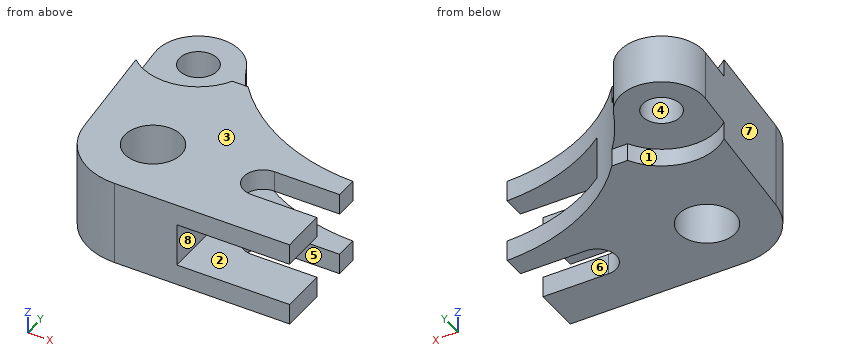
from build123d import *

# Parameters (mm, degrees)
ESQUISSE1_R                  = 9.5
ESQUISSE1_R_2                = 6.35
BOSS_EXTRU_1_DEPTH           = 14.25
ENL_V_MAT_EXTRU_1_DEPTH      = 6
ENL_V_MAT_EXTRU_2_DEPTH      = 7.25
ENL_V_MAT_EXTRU_2_DEPTH_BACK = 7.25


with BuildPart() as part:
    # Esquisse1 → Boss.-Extru.1 (new, symmetric)
    with BuildSketch(Plane.XY):
        with BuildLine():
            Line((-26.61523279, 45.963348263), (-21.894870769, -2.148169925))
            ThreePointArc((-21.894870769, -2.148169925), (-14.777351956, -16.298155392), (0, -22))
            Line((0, -22), (59, -22))
            Line((59, -22), (59, -6.5))
            Line((59, -6.5), (37, -6.5))
            ThreePointArc((37, -6.5), (30.5, 0), (37, 6.5))
            Line((37, 6.5), (59, 6.5))
            Line((59, 6.5), (59, 14))
            ThreePointArc((59, 14), (23.937620364, 25.155899787), (0.053417306, 53.144636986))
            ThreePointArc((0.053417306, 53.144636986), (-16.322360933, 60.848824799), (-26.61523279, 45.963348263))
        make_face()
        with Locations(Location((0, 0, 0), (0, 0, 180))):
            Circle(ESQUISSE1_R, mode=Mode.SUBTRACT)
        with Locations(Location((-12.68213321, 47.330365488, 0), (0, 0, 180))):
            Circle(ESQUISSE1_R_2, mode=Mode.SUBTRACT)
    extrude(amount=BOSS_EXTRU_1_DEPTH, both=True)

    # Esquisse2 → Enlèv. mat.-Extru.1 (cut)
    with BuildSketch(Plane.XY.offset(14.25)):
        with BuildLine():
            Line((4.051067321, 38.330365488), (9.321809703, 38.330365488))
            ThreePointArc((9.321809703, 38.330365488), (4.202566317, 45.434036591), (0.053417306, 53.144636986))
            ThreePointArc((0.053417306, 53.144636986), (-16.322360933, 60.848824799), (-26.61523279, 45.963348263))
            Line((-26.61523279, 45.963348263), (-25.360971776, 33.179497931))
            ThreePointArc((-25.360971776, 33.179497931), (-9.404585059, 28.615193084), (4.051067321, 38.330365488))
        make_face()
    enl_v_mat_extru_1 = extrude(amount=-ENL_V_MAT_EXTRU_1_DEPTH, mode=Mode.SUBTRACT)

    # Symétrie1: Enlèv. mat.-Extru.1 across plane
    add(enl_v_mat_extru_1.mirror(Plane.XY), mode=Mode.SUBTRACT)

    # Esquisse3 → Enlèv. mat.-Extru.2 (cut, two sides: drawn at the far end of the back side and taken through both)
    with BuildSketch(Plane.XY.offset(-ENL_V_MAT_EXTRU_2_DEPTH_BACK)):
        with BuildLine():
            Line((21, -22), (21, 27.222240802))
            ThreePointArc((21, 27.222240802), (38.984037644, 17.691299917), (59, 14))
            Line((59, 14), (59, -22))
            Line((59, -22), (21, -22))
        make_face()
    extrude(amount=ENL_V_MAT_EXTRU_2_DEPTH + ENL_V_MAT_EXTRU_2_DEPTH_BACK, mode=Mode.SUBTRACT)


solid = part.part
Check sheet for the modelled part. Datum: model origin and axes. Units: mm. Face numbers are marked on the shaded views. A direction names the side the tool comes from. Give positions to 0.01 mm unless a question says otherwise; leave off trailing zeros. Loops run counter-clockwise (first coordinate to the right, second up) from the corner with the lowest first, then second, coordinate; pieces in that order, holes last. Notation, with made-up numbers: M 15,-21.5 L 54,-21.5 A27 cw 54,3.5 Z; hole C 23.25,-20 d2. An arc over 180 degrees is marked long. Use a Markdown table: item, result. Add a question column.
Q1. Go/stop test with flat-tipped pins: pin 1 (4.5 mm diameter, centred on y = 0.5, z = -0.5, fed in from +X); pin 2 (6 mm diameter, centred on x = 7, z = -10.5, fed in from +Y); pin 3 (2 mm diameter, centred on x = -10.5, y = 35, fed in from -Z); pin 4 (3 mm diameter, centred on x = 31.5, y = 23, fed in from -Z). Record where each tip stops, or that it passes through.
Q2. Tool access check on the marked faces 1, 2, 3, 4 and 5. Record the directions out of +Z, -Z, +X, -X, +Y, -Y that give a thin tool (end or side, any length) a straight path to the whole face; none if there is none.
Q3. Sectioned sample at A-A, the plane x = 53. Record the cut outline in (y, z).
Q4. Sectioned sample at C-C, the plane x = -15. Record the cut outline in (y, z).
Q5. Mould release check, pull along Y, two halves, no side actions. Record for the marked faces 6, 7 and 8: pulls with the +Y half, pulls with the -Y half, needs draft (parallel to the pull), parting line crosses it, or undercut.
Q6. Sectioned sample at B-B, the plane y = 0. Record the cut outline in (x, z).
Q7. Scan lines: line 1 along Z through (x, y) = (23, -14); line 2 along Y through (x, z) = (0, 5); line 3 along Y through (x, z) = (47, -12.25). Record each from-to range of solid material in increasing order. Write a range as [from, to].
Q8. Sectioned sample at D-D, the plane z = 1.75. Record the cut outline in (x, y), then the cut area to 3 significant figures.
Verdict:
| question | item | result |
|---|---|---|
| 1 | pin 1 | x = 21 |
| 1 | pin 2 | y = 44.17 |
| 1 | pin 3 | z = -8.25 |
| 1 | pin 4 | through |
| 2 | face 1 | -Z, +Y |
| 2 | face 2 | +X, +Y, -Y |
| 2 | face 3 | +Z, +X, -X, +Y, -Y |
| 2 | face 4 | +Z, -Z |
| 2 | face 5 | +Z, -Z, +X |
| 3 | outline | M -22,-14.25 L -6.5,-14.25 L -6.5,-7.25 L -22,-7.25 Z; M -22,7.25 L -6.5,7.25 L -6.5,14.25 L -22,14.25 Z; M 6.5,-14.25 L 14.45,-14.25 L 14.45,-7.25 L 6.5,-7.25 Z; M 6.5,7.25 L 14.45,7.25 L 14.45,14.25 L 6.5,14.25 Z |
| 4 | outline | M -16.09,-14.25 L 28.47,-14.25 L 28.47,-8.25 L 41.42,-8.25 L 41.42,8.25 L 28.47,8.25 L 28.47,14.25 L -16.09,14.25 Z; M 53.24,-8.25 L 61.14,-8.25 L 61.14,8.25 L 53.24,8.25 Z |
| 5 | face 6 | undercut |
| 5 | face 7 | pulls with the -Y half |
| 5 | face 8 | needs draft |
| 6 | outline | M -22.11,-14.25 L -9.5,-14.25 L -9.5,14.25 L -22.11,14.25 Z; M 9.5,-14.25 L 30.5,-14.25 L 30.5,-7.25 L 21,-7.25 L 21,7.25 L 30.5,7.25 L 30.5,14.25 L 9.5,14.25 Z |
| 7 | line 1 | [-14.25, -7.25], [7.25, 14.25] |
| 7 | line 2 | [-22, -9.5], [9.5, 53.26] |
| 7 | line 3 | [-22, -6.5], [6.5, 15.45] |
| 8 | outline | M -26.62,45.96 L -21.89,-2.15 A22 ccw 0,-22 L 21,-22 L 21,27.22 A67 cw 0.05,53.14 A14 ccw Z; hole C -12.68,47.33 d12.7; hole C 0,0 d19 |
| 8 | area | 2,690 mm^2 |
